```python
from build123d import *

# Parameters (mm, degrees)
BOSS_EXTRUDE1_DEPTH     = 5.3
CIRPATTERN1_COUNT       = 10
FILLET1_R               = 0.2
FILLET3_R               = 0.2
SKETCH2_R               = 10
SKETCH2_R_2             = 4.05
BOSS_EXTRUDE2_DEPTH     = 16.7
CUT_EXTRUDE1_DEPTH      = 29.341701561
CUT_EXTRUDE1_DEPTH_BACK = 29.341701561
SKETCH2_2_R             = 4.05
SKETCH3_R               = 17.5
BOSS_EXTRUDE3_DEPTH     = 10
SKETCH3_3_R             = 17.5
CUT_EXTRUDE2_DEPTH      = 34.11344138


with BuildPart() as part:
    # Sketch1 → Boss-Extrude1 (new body)
    with BuildSketch(Plane(origin=(0, 0, 0), x_dir=(0, 0, -1), z_dir=(1, 0, 0))):
        with BuildLine():
            Line((0, 0), (0, 16.75))
            Line((0, 16.75), (1.800167381, 14.035023954))
            ThreePointArc((1.800167381, 14.035023954), (3.754556482, 11.555336673), (6.793214092, 12.412684734))
            Line((6.793214092, 12.412684734), (9.845402976, 13.551034656))
            Line((9.845402976, 13.551034656), (0, 0))
        make_face()
    boss_extrude1 = extrude(amount=BOSS_EXTRUDE1_DEPTH)

    # CirPattern1: Boss-Extrude1 ×10 about axis
    cirpattern1_axis = Axis((0, 0, 0), (1, 0, 0))
    for i in range(1, CIRPATTERN1_COUNT):
        add(boss_extrude1.rotate(cirpattern1_axis, i * 360 / CIRPATTERN1_COUNT))

    # Fillet1
    fillet1_edges = [part.edges().sort_by_distance(p)[0] for p in [
        (2.65, 16.75, 0),
    ]]
    fillet(fillet1_edges, radius=FILLET1_R)

    # Fillet3
    fillet3_edges = [part.edges().sort_by_distance(p)[0] for p in [
        (2.65, 13.551034656, -9.845402976),
        (2.65, 13.551034656, 9.845402976),
        (2.65, 5.176034656, 15.930196648),
        (2.65, -5.176034656, 15.930196648),
        (2.65, -13.551034656, 9.845402976),
        (2.65, -16.75, 0),
        (2.65, -13.551034656, -9.845402976),
        (2.65, -5.176034656, -15.930196648),
        (2.65, 5.176034656, -15.930196648),
    ]]
    fillet(fillet3_edges, radius=FILLET3_R)

    # Sketch2 → Boss-Extrude2 (add)
    with BuildSketch(Plane.ZY):
        with Locations(Location((0, 0, 0), (0, 0, 180))):
            Circle(SKETCH2_R)
        Circle(SKETCH2_R_2, mode=Mode.SUBTRACT)
    extrude(amount=BOSS_EXTRUDE2_DEPTH)

    # Sketch2_2 → Cut-Extrude1 (cut, two sides: drawn at the far end of the back side and taken through both)
    with BuildSketch(Plane.ZY.offset(-CUT_EXTRUDE1_DEPTH_BACK)):
        Circle(SKETCH2_2_R)
    extrude(amount=CUT_EXTRUDE1_DEPTH + CUT_EXTRUDE1_DEPTH_BACK, mode=Mode.SUBTRACT)

    # Sketch3_3 → Cut-Extrude2 (cut, through all)
    with BuildSketch(Plane(origin=(5.3, 0, 0), x_dir=(0, 0, -1), z_dir=(1, 0, 0))):
        Circle(SKETCH3_3_R)
    extrude(amount=-CUT_EXTRUDE2_DEPTH, mode=Mode.SUBTRACT)


with BuildPart() as body_2:
    # Sketch3 → Boss-Extrude3 (new body)
    with BuildSketch(Plane(origin=(5.3, 0, 0), x_dir=(0, 0, -1), z_dir=(1, 0, 0))):
        Circle(SKETCH3_R)
        with BuildLine():
            Line((6.793214092, 12.412684734), (9.562783501, 13.445628382))
            ThreePointArc((9.562783501, 13.445628382), (9.750230279, 13.420040677), (9.832489873, 13.249675233))
            Line((9.832489873, 13.249675233), (9.7059461, 10.296461057))
            ThreePointArc((9.7059461, 10.296461057), (9.829556482, 7.141590815), (12.791818675, 6.049121837))
            Line((12.791818675, 6.049121837), (15.639596437, 5.256878748))
            ThreePointArc((15.639596437, 5.256878748), (15.77620399, 5.125999408), (15.742615104, 4.939819893))
            Line((15.742615104, 4.939819893), (13.904383302, 2.625))
            ThreePointArc((13.904383302, 2.625), (12.15, 0), (13.904383302, -2.625))
            Line((13.904383302, -2.625), (15.742615104, -4.939819893))
            ThreePointArc((15.742615104, -4.939819893), (15.77620399, -5.125999408), (15.639596437, -5.256878748))
            Line((15.639596437, -5.256878748), (12.791818675, -6.049121837))
            ThreePointArc((12.791818675, -6.049121837), (9.829556482, -7.141590815), (9.7059461, -10.296461057))
            Line((9.7059461, -10.296461057), (9.832489873, -13.249675233))
            ThreePointArc((9.832489873, -13.249675233), (9.750230279, -13.420040677), (9.562783501, -13.445628382))
            Line((9.562783501, -13.445628382), (6.793214092, -12.412684734))
            ThreePointArc((6.793214092, -12.412684734), (3.754556482, -11.555336673), (1.800167381, -14.035023954))
            Line((1.800167381, -14.035023954), (0.166687705, -16.498604974))
            ThreePointArc((0.166687705, -16.498604974), (0, -16.588082537), (-0.166687705, -16.498604974))
            Line((-0.166687705, -16.498604974), (-1.800167381, -14.035023954))
            ThreePointArc((-1.800167381, -14.035023954), (-3.754556482, -11.555336673), (-6.793214092, -12.412684734))
            Line((-6.793214092, -12.412684734), (-9.562783501, -13.445628382))
            ThreePointArc((-9.562783501, -13.445628382), (-9.750230279, -13.420040677), (-9.832489873, -13.249675233))
            Line((-9.832489873, -13.249675233), (-9.7059461, -10.296461057))
            ThreePointArc((-9.7059461, -10.296461057), (-9.829556482, -7.141590815), (-12.791818675, -6.049121837))
            Line((-12.791818675, -6.049121837), (-15.639596437, -5.256878748))
            ThreePointArc((-15.639596437, -5.256878748), (-15.77620399, -5.125999408), (-15.742615104, -4.939819893))
            Line((-15.742615104, -4.939819893), (-13.904383302, -2.625))
            ThreePointArc((-13.904383302, -2.625), (-12.15, 0), (-13.904383302, 2.625))
            Line((-13.904383302, 2.625), (-15.742615104, 4.939819893))
            ThreePointArc((-15.742615104, 4.939819893), (-15.77620399, 5.125999408), (-15.639596437, 5.256878748))
            Line((-15.639596437, 5.256878748), (-12.791818675, 6.049121837))
            ThreePointArc((-12.791818675, 6.049121837), (-9.829556482, 7.141590815), (-9.7059461, 10.296461057))
            Line((-9.7059461, 10.296461057), (-9.832489873, 13.249675233))
            ThreePointArc((-9.832489873, 13.249675233), (-9.750230279, 13.420040677), (-9.562783501, 13.445628382))
            Line((-9.562783501, 13.445628382), (-6.793214092, 12.412684734))
            ThreePointArc((-6.793214092, 12.412684734), (-3.754556482, 11.555336673), (-1.800167381, 14.035023954))
            Line((-1.800167381, 14.035023954), (-0.166687705, 16.498604974))
            ThreePointArc((-0.166687705, 16.498604974), (0, 16.588082537), (0.166687705, 16.498604974))
            Line((0.166687705, 16.498604974), (1.800167381, 14.035023954))
            ThreePointArc((1.800167381, 14.035023954), (3.754556482, 11.555336673), (6.793214092, 12.412684734))
        make_face(mode=Mode.SUBTRACT)
    extrude(amount=BOSS_EXTRUDE3_DEPTH)


solid = body_2.part
```
The model under review builds one solid part; all positions refer to its coordinate system, in mm. A direction names the side the tool comes from. Round coordinates to 2 decimals unless told otherwise and drop trailing zeros. Order: outer loops, then holes, each group sorted by start corner. A loop starts at its lowest first (then second) coordinate and runs counter-clockwise, first axis right, second up.
(1) For P1, Ø1.5, axis at x = 8.5, y = -9, coming from the -Z side; P2, Ø3, axis at x = 11.5, y = 8.5, coming from the -Z side, all flat-tipped, find the tip position at first contact; note any pin that passes through.
Working result:
P1: stops at z = -15.43
P2: stops at z = -16.04
(2) Tool access review of faces 4 (the face through (15.3, -12, 5)), 5 (the face through (10.23, -15.25, -0.995)): name each direction out of +Z, -Z, +X, -X, +Y, -Y from which nothing blocks a thin tool from reaching the whole face with its end or side.
Working result:
face 4: +Z, -Z, +X, +Y, -Y
face 5: +X, -X
(3) Take a section at B-B, the plane z = -10.5. State the section outline as (x, y) points, plus the area to 3 significant figures.
Working result:
outline: (5.3, -14) - (15.3, -14) - (15.3, -6.48) - (5.3, -6.48) - close; (5.3, 6.48) - (15.3, 6.48) - (15.3, 14) - (5.3, 14) - close
area: 150 mm2
(4) Take a section at A-A, the plane y = 0. State the section outline as (x, z) points.
Working result:
outline: (5.3, -17.5) - (15.3, -17.5) - (15.3, -12.15) - (5.3, -12.15) - close; (5.3, 12.15) - (15.3, 12.15) - (15.3, 17.5) - (5.3, 17.5) - close
(5) Wall thickness on L1, parallel to Z at x = 13, y = -12; L2, parallel to Y at x = 8.5, z = 14; L3, parallel to Z at x = 13.75, y = 5: over which ranges is each line inside the solid? List them lowest first.
Working result:
L1: z = -12.74 to -9.78, -6.36 to -2.91, 2.91 to 6.36, 9.78 to 12.74
L2: y = -10.5 to -5.71, -2.75 to 2.75, 5.71 to 10.5
L3: z = -16.77 to -15.78, 15.78 to 16.77
(6) Mouldability with a two-part tool opening along Z and no side actions: class faces 1 (the face through (10.23, -7.18, 9.8)), 2 (the face through (5.3, -12, 5)), 3 (the face through (10.23, -10.648, 13.887)) as released by +Z, released by -Z, zero draft, split by the parting line, or undercut.
Working result:
face 1: undercut
face 2: zero draft
face 3: split by the parting line
